Geometry: final body of the model. Coordinates: model frame, mm. A direction names the side the tool comes from. Coordinates: 2 decimals unless noted, no trailing zeros. Loops run counter-clockwise (first coordinate to the right, second up) from the corner with the lowest first, then second, coordinate; pieces in that order, holes last. Notation, with made-up numbers: (53.25, 31.25) -> (105.25, 31.25) arc R19 ccw to (105.25, 65.25) -> close; hole circle Ø4 at (-2.5, -0.75). An arc over 180 degrees is marked (long way). One line per item, written item: value. Start each with the question number.
from build123d import *

# Parameters (mm, degrees)
SKETCH2_W           = 40
SKETCH2_H           = 40
BOSS_EXTRUDE1_DEPTH = 100
SHELL1_T            = -2.5
SKETCH3_R           = 6
CUT_EXTRUDE1_DEPTH  = 2.5


with BuildPart() as part:
    # Sketch2 → Boss-Extrude1 (new body)
    with BuildSketch(Plane(origin=(0, 0, 0), x_dir=(0, 0, -1), z_dir=(1, 0, 0))):
        with Locations((20, 20)):
            Rectangle(SKETCH2_W, SKETCH2_H)
    extrude(amount=BOSS_EXTRUDE1_DEPTH)

    # Shell1
    shell1_openings = [part.faces().sort_by_distance(p)[0] for p in [
        (100, 20, -20),
        (0, 20, -20),
    ]]
    offset(amount=SHELL1_T, openings=shell1_openings, kind=Kind.INTERSECTION)

    # Sketch3 → Cut-Extrude1 (cut)
    with BuildSketch(Plane(origin=(0, 0, -40), x_dir=(-1, 0, 0), z_dir=(0, 0, -1))):
        with Locations((-50, 20)):
            Circle(SKETCH3_R)
    extrude(amount=-CUT_EXTRUDE1_DEPTH, mode=Mode.SUBTRACT)


solid = part.part
1. Line query: L1, parallel to Z at x = 45, y = 13; L2, parallel to Y at x = 50, z = -38; L3, parallel to Y at x = 31, z = -23.5. Output: solid intervals per line, ascending. Write a range as [from, to].
2. Section D-D on y = 3.5. Return the cut outline in (x, z).
3. Draft query along Z for faces 4 (the face through (49, 0, -20)), 5 (the face through (49, 2.5, -20)), 6 (the face through (49, 20, 0)), 7 (the face through (49, 29, -40)). Return one class per face: released by +Z, released by -Z, zero draft, split by the parting line, or undercut.
4. Section A-A on y = 20. Return the cut outline in (x, z).
5. Section C-C on z = -25.5. Return the cut outline in (x, y), plus the area to 3 significant figures.
6. Pin query (flat end, axial travel): pin 1 Ø5 at (x, y) = (22, 28) entering from +Z. Return the tip coordinate at first contact, or that it passes through.
7. Section B-B on x = 75.5. Return the cut outline in (y, z).
8. Set-up query: faces 1 (the face through (56, 20, -39)), 2 (the face through (100, 20, -2)), 3 (the face through (49, 28, -37.5)). Return all of +Z, -Z, +X, -X, +Y, -Y with unobstructed straight access to the full face (end or side cutting, diameter ignored); none if empty.
Checks:
1. L1: [-40, -37.5], [-2.5, 0]
1. L2: [0, 14], [26, 40]
1. L3: [0, 2.5], [37.5, 40]
2. outline: (0, -40) -> (100, -40) -> (100, -37.5) -> (0, -37.5) -> close; (0, -2.5) -> (100, -2.5) -> (100, 0) -> (0, 0) -> close
3. face 4: zero draft
3. face 5: undercut
3. face 6: released by +Z
3. face 7: released by -Z
4. outline: (0, -40) -> (44, -40) -> (44, -37.5) -> (0, -37.5) -> close; (0, -2.5) -> (100, -2.5) -> (100, 0) -> (0, 0) -> close; (56, -40) -> (100, -40) -> (100, -37.5) -> (56, -37.5) -> close
5. outline: (0, 0) -> (100, 0) -> (100, 2.5) -> (0, 2.5) -> close; (0, 37.5) -> (100, 37.5) -> (100, 40) -> (0, 40) -> close
5. area: 500 mm²
6. pin 1: z = 0
7. outline: (0, -40) -> (40, -40) -> (40, 0) -> (0, 0) -> close; hole (2.5, -37.5) -> (37.5, -37.5) -> (37.5, -2.5) -> (2.5, -2.5) -> close
8. face 1: -Z
8. face 2: +Z, -Z, +X, +Y, -Y
8. face 3: +X, -X
